Could you check a few things on this model? Use its own coordinates, in mm. A direction names the side the tool comes from. Give positions to 0.01 mm unless a question says otherwise; leave off trailing zeros. Write each loop counter-clockwise with the first axis right and the second up, starting at its lowest first coordinate (ties: lowest second). Pieces come first, ordered by that corner, then holes. Notation, with made-up numbers: (-26, 64.25) -> (-21, 64.25) arc R26 cw to (-21, 100.25) -> close; hole circle Ø1 at (42, 85). An arc over 180 degrees is marked (long way). One line per question, with ' | ' between items.
from build123d import *

# Parameters (mm, degrees)
SKETCH1_W                  = 26.543
SKETCH1_H                  = 68.58
SKETCH1_W_2                = 21.463
SKETCH1_H_2                = 63.5
BOSS_EXTRUDE1_DEPTH        = 17.78
SKETCH1_4_W                = 26.543
SKETCH1_4_H                = 68.58
SKETCH1_4_W_2              = 21.463
SKETCH1_4_H_2              = 63.5
BOSS_EXTRUDE2_DEPTH        = 6.35
SKETCH2_W                  = 12.319
SKETCH2_H                  = 18.415
CUT_EXTRUDE1_DEPTH         = 3.175
SKETCH3_W                  = 21.463
SKETCH3_H                  = 12.7
BOSS_EXTRUDE3_DEPTH        = 5.08
SKETCH4_R                  = 2.1336
CUT_EXTRUDE2_DEPTH         = 72.405291183
FILLET1_R                  = 2.54
F_10_32_TAPPED_HOLE1_D     = 4.0386
F_10_32_TAPPED_HOLE1_DEPTH = 12.0396
F_10_32_TAPPED_HOLE1_TIP   = 1.213317848


with BuildPart() as part:
    # Sketch1 → Boss-Extrude1 (new body)
    with BuildSketch(Plane(origin=(0, 0, 0), x_dir=(1, 0, 0), z_dir=(0, 1, 0))):
        with Locations((10.7315, 31.75)):
            Rectangle(SKETCH1_W, SKETCH1_H)
        with Locations((10.7315, 31.75)):
            Rectangle(SKETCH1_W_2, SKETCH1_H_2, mode=Mode.SUBTRACT)
    extrude(amount=BOSS_EXTRUDE1_DEPTH)

    # Sketch1_4 → Boss-Extrude2 (add)
    with BuildSketch(Plane(origin=(0, 0, 0), x_dir=(1, 0, 0), z_dir=(0, 1, 0))):
        with Locations((10.7315, 31.75)):
            Rectangle(SKETCH1_4_W, SKETCH1_4_H)
        with Locations((10.7315, 31.75)):
            Rectangle(SKETCH1_4_W_2, SKETCH1_4_H_2, mode=Mode.SUBTRACT)
        with Locations((10.7315, 31.75)):
            Rectangle(SKETCH1_4_W_2, SKETCH1_4_H_2)
    extrude(amount=-BOSS_EXTRUDE2_DEPTH)

    # Sketch2 → Cut-Extrude1 (cut)
    with BuildSketch(Plane(origin=(0, 0, -66.04), x_dir=(-1, 0, 0), z_dir=(0, 0, -1))):
        with Locations((-9.2075, 8.5725)):
            Rectangle(SKETCH2_W, SKETCH2_H)
    extrude(amount=-CUT_EXTRUDE1_DEPTH, mode=Mode.SUBTRACT)

    # Sketch3 → Boss-Extrude3 (add)
    with BuildSketch(Plane(origin=(0, 0, 0), x_dir=(1, 0, 0), z_dir=(0, 1, 0))):
        with Locations((10.7315, 6.35)):
            Rectangle(SKETCH3_W, SKETCH3_H)
    extrude(amount=BOSS_EXTRUDE3_DEPTH)

    # Sketch4 → Cut-Extrude2 (cut, through all)
    with BuildSketch(Plane(origin=(0, 5.08, 0), x_dir=(1, 0, 0), z_dir=(0, 1, 0))):
        with Locations(Location((9.2315, 4.447556381, 0), (0, 0, 270))):
            Circle(SKETCH4_R)
    extrude(amount=-CUT_EXTRUDE2_DEPTH, mode=Mode.SUBTRACT)

    # Fillet1
    fillet1_edges = [part.edges().sort_by_distance(p)[0] for p in [
        (-2.54, 5.715, -66.04),
        (24.003, 5.715, -66.04),
        (24.003, 5.715, 2.54),
        (-2.54, 5.715, 2.54),
        (10.7315, 5.08, -12.7),
    ]]
    fillet(fillet1_edges, radius=FILLET1_R)

    # 10-32 Tapped Hole1
    with Locations(Plane(origin=(0, 0, 0), x_dir=(1, 0, 0), z_dir=(0, 1, 0))):
        with Locations((3.81, 16.51), (17.653, 16.51), (17.653, 59.69), (3.81, 59.69)):
            Hole(F_10_32_TAPPED_HOLE1_D / 2, depth=F_10_32_TAPPED_HOLE1_DEPTH)
            with Locations((0, 0, -(F_10_32_TAPPED_HOLE1_DEPTH + F_10_32_TAPPED_HOLE1_TIP / 2))):  # 118° drill point
                Cone(0, F_10_32_TAPPED_HOLE1_D / 2, F_10_32_TAPPED_HOLE1_TIP, mode=Mode.SUBTRACT)


solid = part.part
Q1. Imagine slicing it at B-B on z = -16.51. Please give me the cut outline in (x, y).
Answer below:
outline: (-2.54, -6.35) -> (1.79, -6.35) -> (1.79, 0) -> (0, 0) -> (0, 17.78) -> (-2.54, 17.78) -> close; (5.83, -6.35) -> (15.63, -6.35) -> (15.63, 0) -> (5.83, 0) -> close; (19.67, -6.35) -> (24, -6.35) -> (24, 17.78) -> (21.46, 17.78) -> (21.46, 0) -> (19.67, 0) -> close
Q2. Imagine slicing it at D-D on y = 10.5. Please give me the cut outline in (x, z), and give its area (3 significant figures).
Answer below:
outline: (-2.54, -63.5) arc R2.54 ccw to (0, -66.04) -> (3.05, -66.04) -> (3.05, -63.5) -> (0, -63.5) -> (0, 0) -> (21.46, 0) -> (21.46, -63.5) -> (15.37, -63.5) -> (15.37, -66.04) -> (21.46, -66.04) arc R2.54 ccw to (24, -63.5) -> (24, 0) arc R2.54 ccw to (21.46, 2.54) -> (0, 2.54) arc R2.54 ccw to (-2.54, 0) -> close | area: 421 mm^2
Q3. On a 3-axis mill with a long thin cutter (end or side, diameter ignored), from which of +Z, -Z, +X, -X, +Y, -Y can I reach the whole of each face in a straight line? I mean faces 1 (the flat face through (3.048, 8, -65)), 2 (the flat face through (0, 9, -31)), 3 (the flat face through (-2.54, 6, -31)). Say none if no direction works.
Answer below:
face 1: -Z, +Y | face 2: +Y | face 3: +Z, -Z, -X, +Y, -Y
Q4. Imagine slicing it at A-A on x = 3.81. Please give me the cut outline in (y, z) (3 decimals), and give its area (3 significant figures).
Answer below:
outline: (-6.35, -66.04) -> (-0.635, -66.04) -> (-0.635, -62.865) -> (0, -62.865) -> (0, -61.709) -> (-6.35, -61.709) -> close; (-6.35, -57.671) -> (0, -57.671) -> (0, -18.529) -> (-6.35, -18.529) -> close; (-6.35, -14.491) -> (0, -14.491) -> (0, -12.7) -> (2.54, -12.7) arc R2.54 ccw to (5.08, -10.16) -> (5.08, 0) -> (17.78, 0) -> (17.78, 2.54) -> (-6.35, 2.54) -> close | area: 490 mm^2
Q5. If I drill on line 1 along Z through (x, y) = (3.81, -3); line 2 along X through (y, z) = (-3.75, -16.51); line 3 along X through (y, z) = (9, -13), over which ranges is the centre line in solid material (lowest first)?
Answer below:
line 1: z = -66.04 to -61.71, -57.67 to -18.53, -14.49 to 2.54 | line 2: x = -2.54 to 1.79, 5.83 to 15.63, 19.67 to 24 | line 3: x = -2.54 to 0, 21.46 to 24
Q6. If we mould it in two halves opening along Z, with no side actions, what happens to faces 4 (the flat face through (15.367, 8, -65)), 5 (the cylindrical face through (19.255, -3.219, -58.461)), 6 (the cylindrical face through (23.279, 5.884, 1.776))? For each: +Z half, -Z half, draft (parallel to the pull), parting line (faces both ways), or undercut.
Answer below:
face 4: draft | face 5: undercut | face 6: +Z half
Q7. Will these pins go through, and if not, where does the flat tip stop? pin 1 (5 mm diameter, centred on x = 13, z = -3, fed in from +Y); pin 2 (1.6 mm diameter, centred on y = 11, z = -64.5, fed in from +X); pin 3 (3 mm diameter, centred on x = 3.81, z = -16.51, fed in from -Y); pin 4 (4 mm diameter, centred on x = 8.5, y = 14, fed in from -Z).
Answer below:
pin 1: stops at y = 5.08 | pin 2: stops at x = 24 | pin 3: passes through | pin 4: stops at z = 0
Q8. Imagine slicing it at C-C on z = -43.5. Please give me the cut outline in (x, y), and give its area (3 significant figures).
Answer below:
outline: (-2.54, -6.35) -> (24, -6.35) -> (24, 17.78) -> (21.46, 17.78) -> (21.46, 0) -> (0, 0) -> (0, 17.78) -> (-2.54, 17.78) -> close | area: 259 mm^2
